Check sheet for the drawn part. Datum: minimum x, y, z corner. Units: mm. Coordinates: 2 decimals unless noted, no trailing zeros. Loops run counter-clockwise (first coordinate to the right, second up) from the corner with the lowest first, then second, coordinate; pieces in that order, holes last.
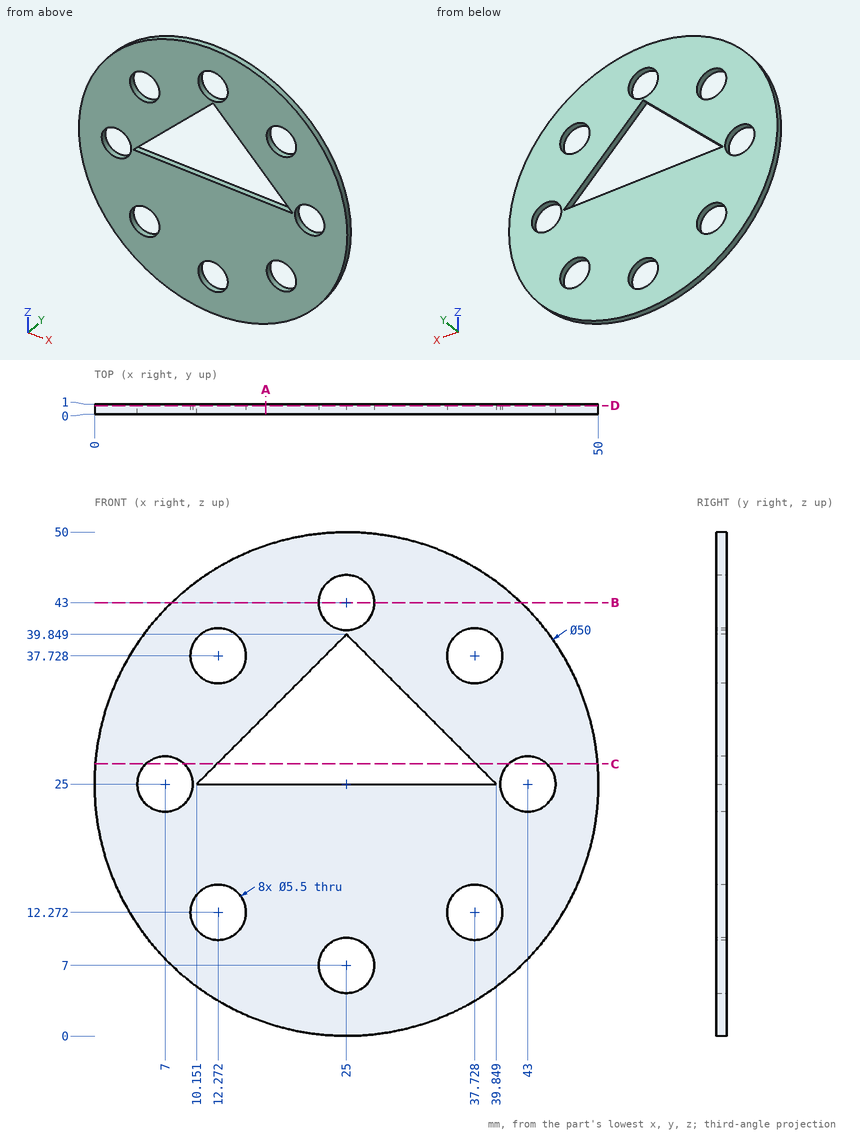
1) Section check B-B on z = 43. Enter the section's corners in (x, y).
Answer sheet:
outline: (7.65, 0) - (22.25, 0) - (22.25, 1) - (7.65, 1) - close; (27.75, 0) - (42.35, 0) - (42.35, 1) - (27.75, 1) - close
2) Section check A-A on x = 17. Enter the section's corners in (y, z) (1 decimal).
Answer sheet:
outline: (0, 1.3) - (1, 1.3) - (1, 25) - (0, 25) - close; (0, 31.8) - (1, 31.8) - (1, 48.7) - (0, 48.7) - close
3) Section check D-D on y = 0.85. Give the number of separate pieces and of enclosed holes in the cut face, plus the area to 3 significant figures.
Answer sheet:
separate pieces: 1
enclosed holes: 9
area: 1,550 mm2
4) Depth check by flat-ended pin: pin 1 (0.5 mm diameter, centred on x = 23, y = 0.5, fed in from +Z); pin 2 (5 mm diameter, centred on x = 37.73, z = 12.27, fed in from -Y). Enter the tip coordinate at first touch or a pass-through.
Answer sheet:
pin 1: stops at z = 49.94
pin 2: passes through
5) Scan lines: line 1 (X direction, y = 0.65, z = 26); line 2 (Z direction, x = 11.5, y = 0.2); line 3 (X direction, y = 0.55, z = 13.5). Record each from-to range of solid material in increasing order.
Answer sheet:
line 1: x = 0.02 to 4.44, 9.56 to 11.15, 38.85 to 40.44, 45.56 to 49.98
line 2: z = 3.96 to 9.63, 14.91 to 25, 26.35 to 35.09, 40.37 to 46.04
line 3: x = 2.8 to 9.81, 14.73 to 35.27, 40.19 to 47.2
6) Section check C-C on z = 27. Enter the section's corners in (x, y), plus the area to 3 significant figures.
Answer sheet:
outline: (0.08, 0) - (5.11, 0) - (5.11, 1) - (0.08, 1) - close; (8.89, 0) - (12.15, 0) - (12.15, 1) - (8.89, 1) - close; (37.85, 0) - (41.11, 0) - (41.11, 1) - (37.85, 1) - close; (44.89, 0) - (49.92, 0) - (49.92, 1) - (44.89, 1) - close
area: 16.6 mm2
